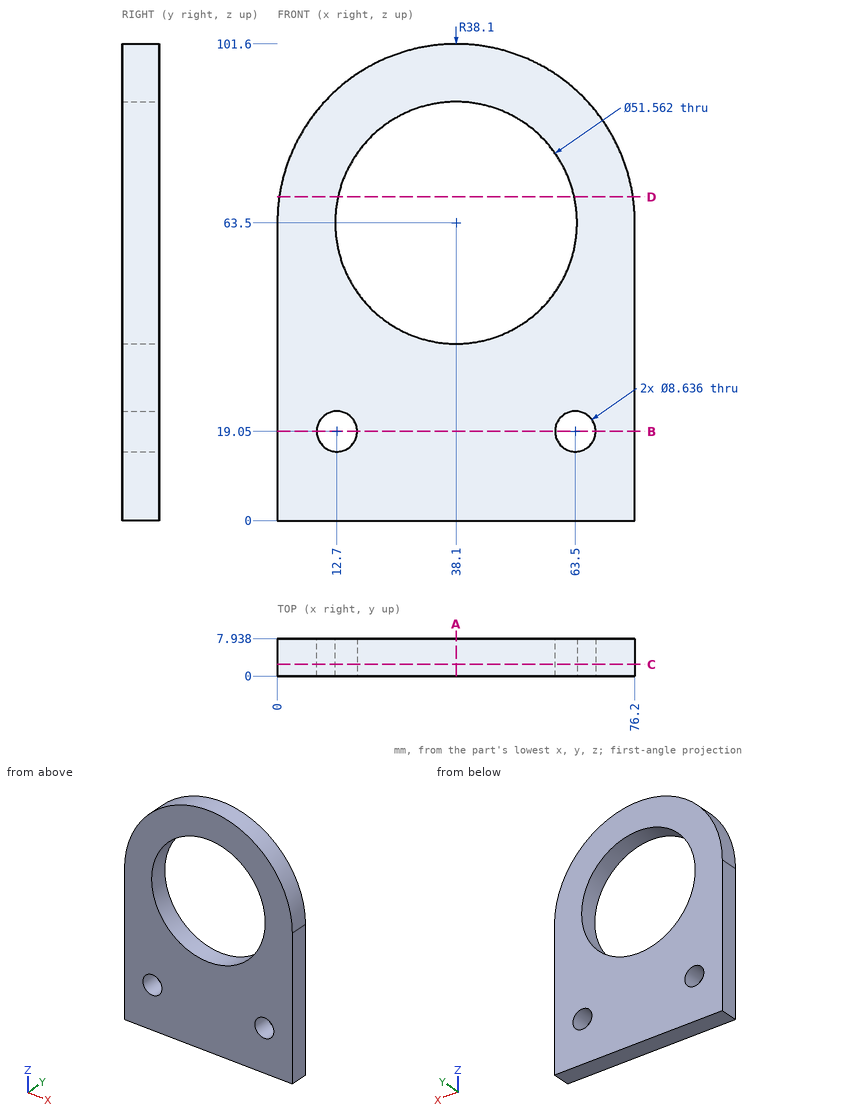
Here's the drawing with two shaded views (mm, measured from the low corner). I have some questions. Coordinates: 2 decimals unless noted, no trailing zeros. Order: outer loops, then holes, each group sorted by start corner. A loop starts at its lowest first (then second) coordinate and runs counter-clockwise, first axis right, second up. Notation, with made-up numbers: M 23.25,2 L 34.25,2 A11 cw 34.25,23 Z; hole C -15.75,3 d1. An arc over 180 degrees is marked long. Write item = value, one per line.
(1) Suppose I cut it at B-B on z = 19.05. Please give me the cut outline in (x, y), plus the area to 3 significant figures.
Results are:
outline = M 0,0 L 8.38,0 L 8.38,7.94 L 0,7.94 Z; M 17.02,0 L 59.18,0 L 59.18,7.94 L 17.02,7.94 Z; M 67.82,0 L 76.2,0 L 76.2,7.94 L 67.82,7.94 Z
area = 468 mm2
(2) Suppose I cut it at D-D on z = 69. Please give me the cut outline in (x, y).
Results are:
outline = M 0.4,0 L 12.91,0 L 12.91,7.94 L 0.4,7.94 Z; M 63.29,0 L 75.8,0 L 75.8,7.94 L 63.29,7.94 Z
(3) I need wall thicknesses on line 1 along X through (y, z) = (5, 57.5); line 2 along Z through (x, y) = (31, 6) (1 decimal); line 3 along Z through (x, y) = (22, 1.25) (1 decimal). Which ranges of each line are inside material? Lowest first, please. Write a range as [from, to].
Results are:
line_1 = [0, 13.03], [63.17, 76.2]
line_2 = [0, 38.7], [88.3, 100.9]
line_3 = [0, 43.4], [83.6, 98]
(4) Suppose I cut it at A-A on x = 38.1. Please give me the cut outline in (y, z), plus the area to 3 significant figures.
Results are:
outline = M 0,0 L 7.94,0 L 7.94,37.72 L 0,37.72 Z; M 0,89.28 L 7.94,89.28 L 7.94,101.6 L 0,101.6 Z
area = 397 mm2
(5) For pin 1 Ø4 at (x, z) = (45, 39.5) entering from +Y; pin 2 Ø1 at (x, y) = (60, 6) entering from +Z, each with a flat end and sliding along its axis, tell me the tip position at first contact or that it passes through.
Results are:
pin_1 = 7.94
pin_2 = 95.02
(6) Suppose I cut it at C-C on y = 2.5. State how many separate pieces and enclosed holes the cut face has, plus the area to 3 significant figures.
Results are:
separate_pieces = 1
enclosed_holes = 3
area = 4,910 mm2
